Autodesk Inventor part; units mm, degrees
ref_plane "作業平面1" through (13.25, -5, 2) normal (0, 0, 1) x (1, 0, 0)
ref_plane "YZ Plane" through (0, 0, 0) normal (1, 0, 0) x (0, 1, 0)
ref_plane "XZ Plane" through (0, 0, 0) normal (0, 1, 0) x (-1, 0, 0)
sketch "スケッチ1" plane through (0, 0, 0) normal (0, 0, 1) x (1, 0, 0)
  ellipse E0 centre (-0.0006, 2.529) end of major axis (-0.0006, 5.5657) minor radius 3.0367 (2.9994, 3) -> (1.7646, 5) ccw
  line L0 (1.7646, 5) -> (-1.7658, 5)
  ellipse E1 centre (-0.0006, 2.529) end of major axis (-0.0006, 5.5657) minor radius 3.0367 (-1.7658, 5) -> (-3.0006, 3) ccw
  arc A0 (-6.0006, 0) -> (-3.0006, 3) centre (-6.0006, 3) ccw
  line L1 (-6.0006, 0) -> (-13.25, 0)
  line L2 (-13.25, -5) -> (-13.25, 0)
  line L3 (-13.25, -5) -> (13.25, -5)
  line L4 (13.25, 0) -> (13.25, -5)
  line L5 (13.25, 0) -> (5.9994, 0)
  ellipse E2 centre (5.9994, 3) end of major axis (8.9994, 3) minor radius 3 (2.9994, 3) -> (5.9994, 0) ccw
  circle A1 centre (-0.0006, 2.529) radius 1
  point P0 (0, 0)
ref_plane "作業平面1" through (13.25, -5, 2) normal (0, 0, 1) x (1, 0, 0)
extrude "押し出し1" add sketch "スケッチ1" along normal up to surface (2 mm away)
sketch "スケッチ2" plane through (-13.25, -5, 2) normal (0, 0, 1) x (1, 0, 0)
  circle A0 centre (13.2494, 7.529) radius 1
  line L0 (19.2494, 5) -> (26.5, 5)
  ellipse E0 centre (19.2494, 8) end of major axis (16.2494, 8) minor radius 3 (16.2494, 8) -> (19.2494, 5) ccw
  ellipse E1 centre (13.2494, 7.529) end of major axis (13.2494, 10.5657) minor radius 3.0367 (16.2494, 8) -> (15.0146, 10) ccw
  line L1 (11.4842, 10) -> (15.0146, 10)
  ellipse E2 centre (13.2494, 7.529) end of major axis (13.2494, 10.5657) minor radius 3.0367 (11.4842, 10) -> (10.2494, 8) ccw
  arc A1 (7.2494, 5) -> (10.2494, 8) centre (7.2494, 8) ccw
  line L2 (0, 5) -> (7.2494, 5)
  line L3 (0, 0) -> (0, 5)
  line L4 (26.5, 0) -> (0, 0)
  line L5 (26.5, 5) -> (26.5, 0)
  line L6 (26.5, 0) -> (26.25, 0)
  line L7 (26.25, 0) -> (26.25, 5)
  line L8 (26.25, 5) -> (26.5, 5)
  line L9 (26.5, 5) -> (26.5, 0)
  line L10 (0, 0) -> (0.25, 0)
  line L11 (0.25, 0) -> (0.25, 5)
  line L12 (0.25, 5) -> (0, 5)
  line L13 (0, 5) -> (0, 0)
  point P0 (13.25, 5)
  point P1 (0.25, 0)
  point P2 (26.25, 0)
  dimension "d2" = 0.25
  dimension "d3" = 0.25
extrude "押し出し2" cut sketch "スケッチ2" against normal blind 10 contours L0 L5 L4 L7 | L4 L3 L2 L11
ref_plane "作業平面2" through (-13, 0, 2) normal (-1, 0, 0) x (0, -1, 0)
sketch "スケッチ3" plane through (-13, 0, 2) normal (-1, 0, 0) x (0, -1, 0)
  line L0 (-95, -2) -> (-84.0931, 10.235)
  line L1 (-84.0931, 10.235) -> (-10.4333, 10.235)
  line L2 (-10.4333, 10.235) -> (-5, 0)
  line L3 (-5, 0) -> (5, 0)
  line L4 (5, 0) -> (5, -3)
  line L5 (-95, -3) -> (5, -3)
  line L6 (-95, -2) -> (-95, -3)
  line L7 (-11, -11.065) -> (-11, 7.535)
  line L8 (-11, 7.535) -> (-84.5, 7.535)
  line L9 (-5, -2) -> (-5, 0)
  line L10 (-5, -2) -> (-10.5, -2)
  line L11 (-10.5, -2) -> (-10.5, 8.035)
  line L12 (-10.5, 8.035) -> (-12.7452, 8.035)
  line L13 (-12.7452, 8.035) -> (-84.6975, 8.035)
  line L14 (-85, -6.5) -> (-85, -5)
  line L15 (-85, -2) -> (-85, -5)
  line L16 (-85, -2) -> (-85, 8.035)
  line L17 (-85, 8.035) -> (-84.5, 8.035)
  line L18 (-85, -2) -> (-95, -2)
  point P0 (0, -2)
  dimension "d6" = 0.5
  dimension "d7" = 0.5
extrude "押し出し3" add sketch "スケッチ3" against normal up to surface (26 mm away) contours L0 L1 L2 L9 L10 L11 L12 L13 L17 L16 L18
sketch "スケッチ4" plane through (0, 0, 0) normal (0, 0, -1) x (-1, 0, 0)
  circle A0 centre (0.0006, 2.529) radius 1
  line L0 (13, -5) -> (13, 0)
  line L1 (6.0006, 0) -> (13, 0)
  arc A1 (3.0006, 3) -> (6.0006, 0) centre (6.0006, 3) ccw
  ellipse E0 centre (0.0006, 2.529) end of major axis (0.0006, 5.5657) minor radius 3.0367 (3.0006, 3) -> (1.7658, 5) ccw
  line L2 (13, 5) -> (1.7658, 5)
  line L3 (13, 10.5) -> (13, 5)
  line L4 (13, 10.5) -> (-13, 10.5)
  line L5 (-13, 5) -> (-13, 10.5)
  line L6 (-1.7646, 5) -> (-13, 5)
  ellipse E1 centre (0.0006, 2.529) end of major axis (0.0006, 5.5657) minor radius 3.0367 (-1.7646, 5) -> (-2.9994, 3) ccw
  ellipse E2 centre (-5.9994, 3) end of major axis (-2.9994, 3) minor radius 3 (-5.9994, 0) -> (-2.9994, 3) ccw
  line L7 (-13, 0) -> (-5.9994, 0)
  line L8 (-13, 0) -> (-13, -5)
  line L9 (13, -5) -> (-13, -5)
  line L10 (-13, 0) -> (-13, 5)
  line L11 (13, 5) -> (13, 0)
  point P0 (0, 0)
extrude "押し出し4" add sketch "スケッチ4" against normal up to surface (2 mm away) contours L1 A1 E0 L2 L11 | L10 L6 E1 E2 L7
sketch "スケッチ5" plane through (-13, 10.4333, 12.235) normal (0, 0, 1) x (1, 0, 0)
  circle A0 centre (13.7123, 77.0667) radius 1
  circle A1 centre (13.7123, 77.0667) radius 2.5
  point P0 (13, -10.4333)
  dimension "d12" = 5
extrude "押し出し5" cut sketch "スケッチ5" against normal blind 13 contours A0
sketch "スケッチ6" plane through (-13, 10.4333, 12.235) normal (0, 0, 1) x (1, 0, 0)
  circle A0 centre (13.7123, 77.0667) radius 1
  circle A1 centre (13.7123, 77.0667) radius 2.5
  point P0 (13, -10.4333)
  dimension "d15" = 5
extrude "押し出し6" cut sketch "スケッチ6" against normal blind 11 contours A0 | A1
sketch "スケッチ7" plane through (-13, 85, 0) normal (0, -1, 0) x (1, 0, 0)
  line L0 (26, 10.035) -> (26, 0)
  line L1 (13.7123, 10.035) -> (26, 10.035)
  line L2 (13.7123, 10.035) -> (13.7123, 1.235)
  line L3 (0, 10.035) -> (13.7123, 10.035)
  line L4 (0, 0) -> (0, 10.035)
  line L5 (0, 0) -> (26, 0)
  point P0 (13, 0)
extrude "押し出し7" add sketch "スケッチ7" along normal blind 1
fillet "フィレット1" radius 2 2 edges at (0, 10.5, 10.035) (0, 84, 10.035)
equation "\"d7\" = d6"
properties part number "NNfront-huta"
Can you work these out from the model? Positions are in its coordinate system, mm. A direction names the side the tool comes from. Coordinates: 2 decimals unless noted, no trailing zeros. Loops run counter-clockwise (first coordinate to the right, second up) from the corner with the lowest first, then second, coordinate; pieces in that order, holes last.
1) Which directions (+Z, -Z, +X, -X, +Y, -Y) give clear straight access to the entire face, cutting with the end or side of a thin tool? Please do faces 4 (the cylindrical face through (0.17, 85.06, 5.19)), 5 (the flat face through (0, 84, 4)), 6 (the flat face through (0, 0, 2)).
2) Imagine slicing it at A-A on y = 87.5. List the corners of the cut face in (x, z) for me (3 decimals).
3) Thinking about a two-plate mould opening in X: for faces 1 (the flat face through (0, 4, 0)), 2 (the flat face through (1, 86, 1.235)), 3 (the flat face through (13, 53, 11)), which applies, pulls with the +X half, pulls with the -X half, needs draft (parallel to the pull), parting line crosses it, or undercut?
4) Imagine slicing it at B-B on x = -6.75. List the corners of the cut face in (y, z) for me (3 decimals).
5) For pin 1 (13 mm diameter, centred on x = -5.5, y = 48, fed in from -Z) (3 decimals); pin 2 (2 mm diameter, centred on x = -5.5, z = 5.5, fed in from -Y); pin 3 (5 mm diameter, centred on x = 8, z = 3.5, fed in from +Y); pin 4 (1.2 mm diameter, centred on x = 0, y = 2.53, fed in from +Z), each with a flat end and sliding along its axis, tell me the tip position at first contact or that it passes through.
6) Imagine slicing it at C-C on y = 29. List the corners of the cut face in (x, z) for me (3 decimals).
7) I need wall thicknesses on probe 1 along X at (y, z) = (87.5, 0.75); probe 2 along Y at (x, z) = (3, 5.25); probe 3 along Z at (x, y) = (-11.5, 42) (3 decimals). Which ranges of each line are inside material? Lowest first, please.
Completed:
1. face 4: +Z
1. face 5: -Z, +X, -X
1. face 6: +Z, +X, -X, -Y
2. outline: (-13, 0) - (-0.288, 0) - (-0.288, 1.235) - (-1.788, 1.235) - (-1.788, 8.413) - (-13, 8.413) - close; (1.712, 0) - (13, 0) - (13, 8.413) - (3.212, 8.413) - (3.212, 1.235) - (1.712, 1.235) - close
3. face 1: needs draft
3. face 2: undercut
3. face 3: pulls with the +X half
4. outline: (-5, 0) - (10.5, 0) - (10.5, 8.035) arc R2 cw to (12.5, 10.035) - (82, 10.035) arc R2 cw to (84, 8.035) - (84, 0) - (95, 0) - (84.093, 12.235) - (10.433, 12.235) - (5, 2) - (-5, 2) - close
5. pin 1: stops at z = 10.035
5. pin 2: stops at y = 6.33
5. pin 3: stops at y = 94.11
5. pin 4: passes through
6. outline: (-13, 10.035) - (13, 10.035) - (13, 12.235) - (-13, 12.235) - close
7. probe 1: x = -13 to -0.29, 1.71 to 13
7. probe 2: y = 6.73 to 10.5, 84 to 86.49, 88.51 to 90.32
7. probe 3: z = 10.035 to 12.235
